```python
from build123d import *

# Parameters (mm, degrees)
F0_R     = 31.217266
F1_DEPTH = 50.8
F2_DEPTH = 12.7
F4_DEPTH = 38.862
F6_DEPTH = 177.8


with BuildPart() as f1:
    # F0 (on Top) → F1 (new body)
    with BuildSketch(Plane.XY):
        with BuildLine():
            ThreePointArc((27.24497, -47.55269), (68.940098, -38.406733), (87.569511, 0))
            ThreePointArc((87.569511, 0), (69.555113, 37.913842), (28.783381, 47.896017))
            ThreePointArc((28.783381, 47.896017), (-10.233562, 0.788128), (27.24497, -47.55269))
        make_face()
        with Locations((38.664799, 0)):
            Circle(F0_R, mode=Mode.SUBTRACT)
    extrude(amount=F1_DEPTH)

    # F0 (on Top) → F2 (join)
    with BuildSketch(Plane.XY):
        with BuildLine():
            ThreePointArc((27.24497, -47.55269), (-10.233562, 0.788128), (28.783381, 47.896017))
            Line((28.783381, 47.896017), (-75.24436, 47.896017))
            Line((-75.24436, 47.896017), (-75.24436, -41.144535))
            Line((-75.24436, -41.144535), (27.24497, -47.55269))
        make_face()
    extrude(amount=F2_DEPTH)

    # F3 (on face) → F4 (join)
    with BuildSketch(Plane.XY.offset(50.8)):
        with BuildLine():
            ThreePointArc((-10.037816, -4.441411), (-10.239913, 0), (-10.037816, 4.441411))
            Line((-10.037816, 4.441411), (-44.907834, 4.441411))
            Line((-44.907834, 4.441411), (-44.907834, -6.231935))
            Line((-44.907834, -6.231935), (-10.037816, -6.231935))
            Line((-10.037816, -6.231935), (-10.037816, -4.441411))
        make_face()
    extrude(amount=-F4_DEPTH)

    # F5 (on face) → F6 (cut)
    with BuildSketch(Plane.XZ.offset(6.231935)):
        Polygon((-44.907834, 50.8), (-44.907834, 12.7), (-10.037816, 50.8), align=None)
    extrude(amount=-F6_DEPTH, mode=Mode.SUBTRACT)


solid = f1.part
```
The model under review builds one solid part; all positions refer to its coordinate system, in mm. A direction names the side the tool comes from. Coordinates: 2 decimals unless noted, no trailing zeros. Write each loop counter-clockwise with the first axis right and the second up, starting at its lowest first coordinate (ties: lowest second). Pieces come first, ordered by that corner, then holes.
1) Clearance check with flat-ended pins moving along their axes: pin 1 Ø5 at (x, y) = (-32, 33) entering from +Z; pin 2 Ø2 at (x, z) = (1, 17) entering from -Y; pin 3 Ø0.5 at (y, z) = (-5, 38) entering from +X. State where each tip first meets the part, or that it passes through.
2) Machinability: for faces 1 (the face through (-27.7, -1, 31.5)), 2 (the face through (-20, -6.232, 24)), 3 (the face through (-23, 47.896, 6)), 4 (the face through (-19, 4.441, 24)), which of the approach directions +Z, -Z, +X, -X, +Y, -Y give a long, thin tool a straight path to every point of the face, cutting with its end or side? Answer none if there is none.
3) We need section D-D on x = -12.5. State the section outline as (y, z) points, then the cut area to 3 significant figures.
4) We need section B-B on y = -11.5. State the section outline as (x, z) points.
5) The part is to be moulded in two halves that separate along Y. For faces 5 (the face through (-24.717, -44.304, 6.261)), 6 (the face through (68.44, 9.38, 25.04)), 7 (the face through (-36, 11, 12.7)), say which applies: pulls with the +Y half, pulls with the -Y half, needs draft (parallel to the pull), parting line crosses it, or undercut.
6) We need section C-C on z = 43. State the section outline as (x, y) points.
7) To check wall thickness, follow probe 1 along Y at (x, z) = (38.5, 15); probe 2 along Z at (x, y) = (-28, 45.5); probe 3 along X at (y, z) = (-15, 21). State the ranges of each line that lie inside material, in increasing order.
8) We need section A-A on x = 24.5. State the section outline as (y, z) points, then the cut area to 3 significant figures.
Answer list:
1. pin 1: stops at z = 12.7
1. pin 2: stops at y = -32.36
1. pin 3: stops at x = 87.34
2. face 1: +Z, -X, +Y, -Y
2. face 2: +Z, -X, -Y
2. face 3: +Z, -Z, -X, +Y
2. face 4: +Z, -X, +Y
3. outline: (-45.07, 0) - (47.9, 0) - (47.9, 12.7) - (4.44, 12.7) - (4.44, 48.11) - (-6.23, 48.11) - (-6.23, 12.7) - (-45.07, 12.7) - close
3. area: 1,560 mm2
4. outline: (-75.24, 0) - (9.64, 0) - (9.64, 50.8) - (-8.87, 50.8) - (-8.87, 12.7) - (-75.24, 12.7) - close; (67.69, 0) - (86.2, 0) - (86.2, 50.8) - (67.69, 50.8) - close
5. face 5: pulls with the -Y half
5. face 6: undercut
5. face 7: needs draft
6. outline: (-17.18, -6.23) - (-10.04, -6.23) - (-10.04, -4.44) arc R48.9 ccw to (87.57, 0) arc R48.9 ccw to (28.78, 47.9) arc R48.9 ccw to (-10.04, 4.44) - (-17.18, 4.44) - close; hole circle Ø62.43 at (38.66, 0)
7. probe 1: y = -48.9 to -31.22, 31.22 to 48.9
7. probe 2: z = 0 to 12.7
7. probe 3: x = -7.88 to 11.29, 66.04 to 85.21
8. outline: (-47.38, 0) - (-27.82, 0) - (-27.82, 50.8) - (-46.81, 50.8) - (-46.81, 12.7) - (-47.38, 12.7) - close; (27.82, 0) - (47.9, 0) - (47.9, 12.7) - (46.81, 12.7) - (46.81, 50.8) - (27.82, 50.8) - close
8. area: 1,950 mm2
